```python
from build123d import *

# Parameters (mm, degrees)
SKETCH1_W           = 35
SKETCH1_H           = 60
SKETCH1_R           = 12.7
BOSS_EXTRUDE1_DEPTH = 20
FILLET1_R           = 10


with BuildPart() as part:
    # Sketch1 → Boss-Extrude1 (new body)
    with BuildSketch(Plane(origin=(0, 0, 0), x_dir=(1, 0, 0), z_dir=(0, 1, 0))):
        Rectangle(SKETCH1_W, SKETCH1_H)
        Circle(SKETCH1_R, mode=Mode.SUBTRACT)
    extrude(amount=BOSS_EXTRUDE1_DEPTH)

    # Fillet1
    fillet1_edges = [part.edges().sort_by_distance(p)[0] for p in [
        (17.5, 10, 30),
        (-17.5, 10, 30),
        (-17.5, 10, -30),
        (17.5, 10, -30),
    ]]
    fillet(fillet1_edges, radius=FILLET1_R)


solid = part.part
```
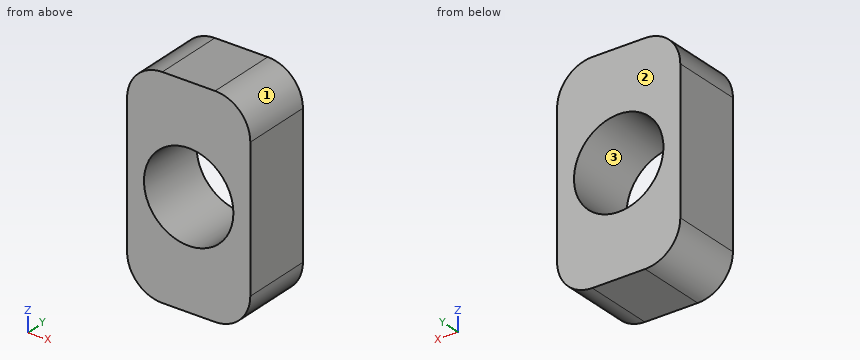
Build history of the part. All positions in model axes, mm. Face numbers are marked on the shaded views. Round coordinates to 2 decimals unless told otherwise and drop trailing zeros. Loops run counter-clockwise (first coordinate to the right, second up) from the corner with the lowest first, then second, coordinate; pieces in that order, holes last.
Item 1: Saw through at A-A (z = 0). List the corners of the cut face in (x, y), then the cut area to 3 significant figures.
Item 2: Saw through at C-C (x = 0). List the corners of the cut face in (y, z), then the cut area to 3 significant figures.
Item 3: Saw through at B-B (y = 8). List the corners of the cut face in (x, z), then the cut area to 3 significant figures.
Item 4: Drill centre lines: line 1 along X through (y, z) = (8.25, 0); line 2 along Z through (x, y) = (0, 12); line 3 along Z through (x, y) = (-5, 13.5). Where is each one in solid material? Low to high.
Item 5: Two-plate mould, pull along Z, no slides. Class the marked faces 1, 2 and 3: released by +Z, released by -Z, zero draft, split by the parting line, or undercut.
Item 6: Saw through at D-D (x = 15.5). List the corners of the cut face in (y, z).
Worked answers:
1. outline: (-17.5, 0) - (-12.7, 0) - (-12.7, 20) - (-17.5, 20) - close; (12.7, 0) - (17.5, 0) - (17.5, 20) - (12.7, 20) - close
1. area: 192 mm2
2. outline: (0, -30) - (20, -30) - (20, -12.7) - (0, -12.7) - close; (0, 12.7) - (20, 12.7) - (20, 30) - (0, 30) - close
2. area: 692 mm2
3. outline: (-17.5, -20) arc R10 ccw to (-7.5, -30) - (7.5, -30) arc R10 ccw to (17.5, -20) - (17.5, 20) arc R10 ccw to (7.5, 30) - (-7.5, 30) arc R10 ccw to (-17.5, 20) - close; hole circle Ø25.4 at (0, 0)
3. area: 1,510 mm2
4. line 1: x = -17.5 to -12.7, 12.7 to 17.5
4. line 2: z = -30 to -12.7, 12.7 to 30
4. line 3: z = -30 to -11.67, 11.67 to 30
5. face 1: released by +Z
5. face 2: zero draft
5. face 3: undercut
6. outline: (0, -26) - (20, -26) - (20, 26) - (0, 26) - close
